Answer from the drawing. Dimensions are ordinates in mm from the lowest x, y and z of the part. A direction names the side the tool comes from. Give positions to 0.01 mm unless a question says otherwise; leave off trailing zeros. Write each loop counter-clockwise with the first axis right and the second up, starting at its lowest first coordinate (ties: lowest second). Pieces come first, ordered by that corner, then holes. Notation, with made-up numbers: M -35,53 L -24,53 A32 cw -24,87 Z; hole C 58,71.25 d4. An arc over 180 degrees is marked long. Write each question's results on one line, items separated by ' | '. Start each with the question number.
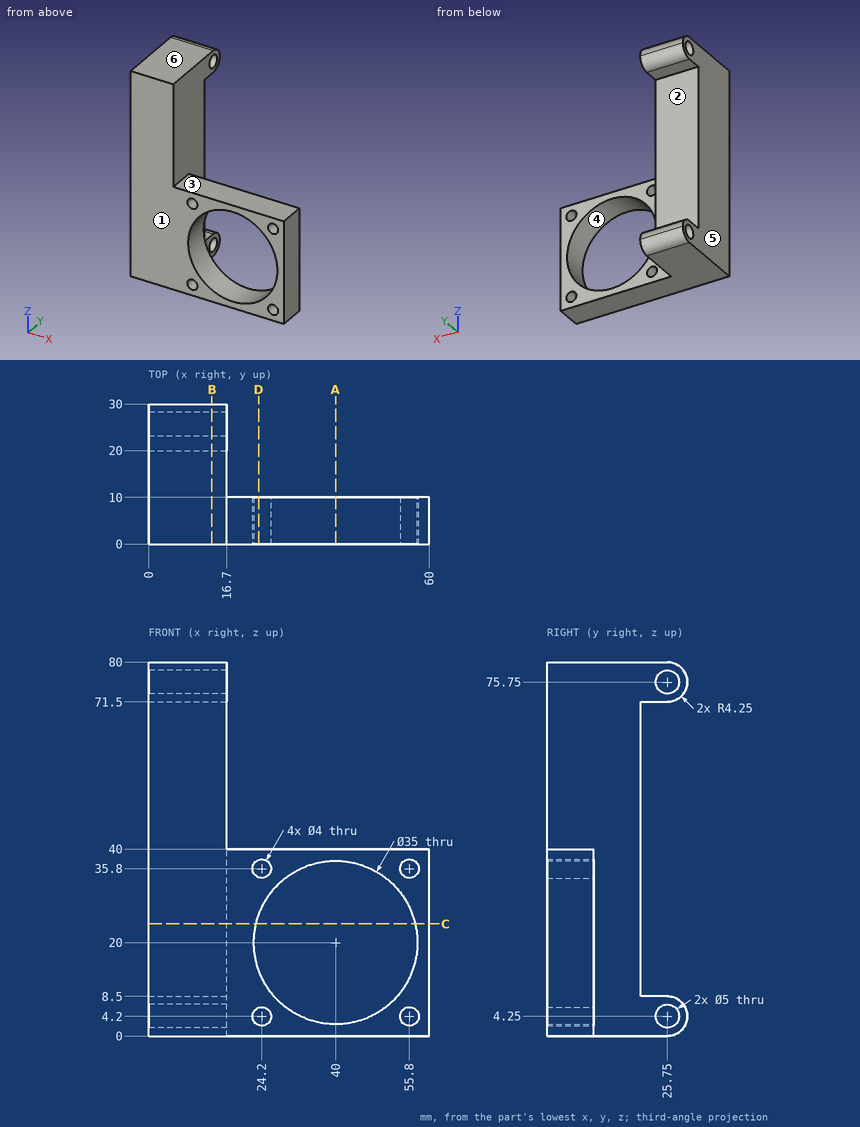
Item 1: Determine the mould class of the marked faces 4, 5 and 6 for opening direction Z: +Z half, -Z half, draft (parallel to the pull), parting line (faces both ways), or undercut.
Item 2: Section C-C, the plane z = 24 is taken. Determine the outline of the cut face in (x, y), then the cut area to 3 significant figures.
Item 3: Section B-B, the plane x = 13.5 is taken. Determine the outline of the cut face in (y, z).
Item 4: Given P1, Ø6, axis at y = 25.75, z = 75.75, coming from the +X side; P2, Ø3.5, axis at x = 55.8, z = 4.2, coming from the -Y side; P3, Ø8.5, axis at x = 11.5, z = 45.5, coming from the +Y side; P4, Ø12, axis at x = 16, z = 63.5, coming from the -Y side, each flat-ended and moving along its own axis, determine where each tip first touches the part or whether it passes through.
Item 5: For the marked faces 1, 2 and 3, determine the directions among +Z, -Z, +X, -X, +Y, -Y from which every point of the face is accessible in a straight line to the end or side of a thin tool.
Item 6: Section A-A, the plane x = 40 is taken. Determine the outline of the cut face in (y, z), then the cut area to 3 significant figures.
Item 7: Straight lines are drawn through the part: line 1 (Z direction, x = 8.25, y = 25.75); line 2 (Z direction, x = 40, y = 5); line 3 (Z direction, x = 24.2, y = 3.25). For each, find the intervals that lie inside material, in ascending order.
Item 8: Section D-D, the plane x = 23.5 is taken. Determine the outline of the cut face in (y, z), then the cut area to 3 significant figures.
Worked out:
1) face 4: undercut | face 5: draft | face 6: +Z half
2) outline: M 0,0 L 22.96,0 L 22.96,10 L 16.7,10 L 16.7,20 L 0,20 Z; M 57.04,0 L 60,0 L 60,10 L 57.04,10 Z | area: 426 mm²
3) outline: M 0,0 L 25.75,0 A4.25 ccw 25.75,8.5 L 20,8.5 L 20,71.5 L 25.75,71.5 A4.25 ccw 25.75,80 L 0,80 Z; hole C 25.75,4.25 d5; hole C 25.75,75.75 d5
4) P1: stops at x = 16.7 | P2: passes through | P3: stops at y = 20 | P4: stops at y = 0
5) face 1: +Z, -Z, +X, -X, -Y | face 2: +X, -X, +Y | face 3: +Z, +X, +Y, -Y
6) outline: M 0,0 L 10,0 L 10,2.5 L 0,2.5 Z; M 0,37.5 L 10,37.5 L 10,40 L 0,40 Z | area: 50.0 mm²
7) line 1: z = 0 to 1.75, 6.75 to 8.5, 71.5 to 73.25, 78.25 to 80 | line 2: z = 0 to 2.5, 37.5 to 40 | line 3: z = 0 to 2.2, 6.2 to 12.48, 27.52 to 33.8, 37.8 to 40
8) outline: M 0,0 L 10,0 L 10,2.33 L 0,2.33 Z; M 0,6.07 L 10,6.07 L 10,14.17 L 0,14.17 Z; M 0,25.83 L 10,25.83 L 10,33.93 L 0,33.93 Z; M 0,37.67 L 10,37.67 L 10,40 L 0,40 Z | area: 208 mm²
